```python
from build123d import *

# Parameters (mm, degrees)
FILLET1_R          = 0.762
CHAMFER1_SIZE      = 0.508
SKETCH2_W          = 1.905
SKETCH2_H          = 1.0795
CUT_EXTRUDE1_DEPTH = 0.5715
CIRPATTERN1_COUNT  = 4


with BuildPart() as part:
    # Sketch1 → Revolve1 (revolve)
    with BuildSketch(Plane.XY, mode=Mode.PRIVATE) as revolve1_sk:
        Polygon((0, 0), (0, 11.43), (2.54, 11.43), (2.54, 8.89), (2.54, 8.636), (2.8321, 8.636), (2.8321, 8.89), (8.255, 8.89), (8.255, 0), align=None)
    revolve(revolve1_sk.sketch.rotate(Axis((0, 0, 0), (0, 1, 0)), 90), axis=Axis((0, 0, 0), (0, 1, 0)))

    # Fillet1
    fillet1_edges = [part.edges().sort_by_distance(p)[0] for p in [
        (0, 8.89, 8.255),
    ]]
    fillet(fillet1_edges, radius=FILLET1_R)

    # Chamfer1
    chamfer1_edges = [part.edges().sort_by_distance(p)[0] for p in [
        (0, 0, 8.255),
    ]]
    chamfer(chamfer1_edges, length=CHAMFER1_SIZE)

    # Sketch2 → Cut-Extrude1 (cut)
    with BuildSketch(Plane.XZ):
        with Locations((5.7785, 0)):
            Rectangle(SKETCH2_W, SKETCH2_H)
    cut_extrude1 = extrude(amount=-CUT_EXTRUDE1_DEPTH, mode=Mode.SUBTRACT)

    # CirPattern1: Cut-Extrude1 ×4 about axis
    cirpattern1_axis = Axis((0, 0, 0), (0, 1, 0))
    for i in range(1, CIRPATTERN1_COUNT):
        add(cut_extrude1.rotate(cirpattern1_axis, i * 360 / CIRPATTERN1_COUNT), mode=Mode.SUBTRACT)


solid = part.part
```
CAD build for the part. Positions are in the model's coordinates, mm. A direction names the side the tool comes from. Give positions to 0.01 mm unless a question says otherwise; leave off trailing zeros. Order: outer loops, then holes, each group sorted by start corner. A loop starts at its lowest first (then second) coordinate and runs counter-clockwise, first axis right, second up.
(1) Flat gauge pins, fed straight in: pin 1 (0.5 mm diameter, centred on x = 0, z = 6, fed in from -Y); pin 2 (0.6 mm diameter, centred on y = 0.5, z = -5.5, fed in from +X); pin 3 (0.6 mm diameter, centred on y = 0.5, z = -5.5, fed in from -X). Where does each tip first touch, or does it go through?
(2) Saw through at C-C, the plane y = 4.25. Give the cut face in (x, z) (3 decimals).
(3) Saw through at D-D, the plane y = 9.75. Give the cut face in (x, z), then the cut area to 3 significant figures.
(4) Drill centre lines: L1, parallel to X at y = 8.75, z = 0; L2, parallel to Y at x = 2.25, z = 3.75; L3, parallel to Y at x = 6, z = 0. Where is each one in solid material? Low to high.
(5) Tool access for faces 1 (the flat face through (-6, 0.572, 0)), 2 (the flat face through (0, 0, 0)), 3 (the flat face through (3, 8.89, 0)): list every direction of +Z, -Z, +X, -X, +Y, -Y with a clear straight run to the whole face (end or side of a thin tool).
(6) Mould opens along X. For faces 4 (the cylindrical face through (7.324, 4.265, -3.809)), 5 (the flat face through (6, 0.572, 0)), 6 (the flat face through (0, 0.572, -6)), 7 (the flat face through (0, 11.43, 0)) say: released by +X, released by -X, zero draft, split by the parting line, or undercut.
Results found:
1. pin 1: stops at y = 0.57
1. pin 2: stops at x = 6.41
1. pin 3: stops at x = -6.41
2. outline: circle Ø16.51 at (0, 0)
3. outline: circle Ø5.08 at (0, 0)
3. area: 20.3 mm2
4. L1: x = -7.93 to -2.83, -2.54 to 2.54, 2.83 to 7.93
4. L2: y = 0 to 8.89
4. L3: y = 0.57 to 8.89
5. face 1: -Y
5. face 2: +Z, -Z, +X, -X, -Y
5. face 3: +Y
6. face 4: split by the parting line
6. face 5: undercut
6. face 6: undercut
6. face 7: zero draft
